```python
from build123d import *

# Parameters (mm, degrees)
F0_W      = 100
F0_H      = 40
F1_DEPTH  = 7
F2_W      = 55
F2_H      = 10
F3_DEPTH  = 8
F4_SIZE   = 3
F5_R      = 2.25
F6_DEPTH  = 18.9
F7_W      = 18
F7_H      = 8
F8_DEPTH  = 3
F9_W      = 55
F9_H      = 10
F10_DEPTH = 1.5
F12_DEPTH = 0.5


# Not quite as in the source:
# - a feature names something its author has since deleted; it is built from what else it names


with BuildPart() as f1:
    # F0 (on Top) → F1 (new body)
    with BuildSketch(Plane.XY):
        with Locations((50, -20)):
            Rectangle(F0_W, F0_H)
    extrude(amount=F1_DEPTH)

    # F2 (on Top) → F3 (cut)
    with BuildSketch(Plane.XY):
        with Locations((50, -20)):
            Rectangle(F2_W, F2_H)
    extrude(amount=F3_DEPTH, mode=Mode.SUBTRACT)

    # F4
    f4_edges = [f1.edges().sort_by_distance(p)[0] for p in [
        (50, -15, 7),
        (22.5, -20, 7),
        (50, -25, 7),
        (77.5, -20, 7),
    ]]
    chamfer(f4_edges, length=F4_SIZE)

    # F5 (on Top) → F6 (cut)
    with BuildSketch(Plane.XY):
        with Locations((12, -35)):
            Circle(F5_R)
        with Locations((31, -35)):
            Circle(F5_R)
        with Locations((50, -35)):
            Circle(F5_R)
        with Locations((69, -35)):
            Circle(F5_R)
        with Locations((88, -35)):
            Circle(F5_R)
        with Locations((95, -28)):
            Circle(F5_R)
        with Locations((95, -12)):
            Circle(F5_R)
        with Locations((88, -5)):
            Circle(F5_R)
        with Locations((69, -5)):
            Circle(F5_R)
        with Locations((50, -5)):
            Circle(F5_R)
        with Locations((31, -5)):
            Circle(F5_R)
        with Locations((12, -5)):
            Circle(F5_R)
        with Locations((5, -12)):
            Circle(F5_R)
        with Locations((5, -28)):
            Circle(F5_R)
    extrude(amount=F6_DEPTH, mode=Mode.SUBTRACT)

    # F7 (on face) → F8 (cut)
    with BuildSketch(Plane(origin=(0, 0, 0), x_dir=(1, 0, 0), z_dir=(0, 0, -1))):
        with Locations((9, 20)):
            Rectangle(F7_W, F7_H)
        with Locations((91, 20)):
            Rectangle(F7_W, F7_H)
    extrude(amount=-F8_DEPTH, mode=Mode.SUBTRACT)

    # F9 (on face) → F10 (cut)
    with BuildSketch(Plane(origin=(0, 0, 0), x_dir=(1, 0, 0), z_dir=(0, 0, -1))):
        Polygon((21, 13.5), (77.5, 13.5), (79, 13.5), (79, 26.5), (21, 26.5), align=None)
        with Locations((50, 20)):
            Rectangle(F9_W, F9_H, mode=Mode.SUBTRACT)
    extrude(amount=-F10_DEPTH, mode=Mode.SUBTRACT)

    # F11 (on face) → F12 (cut)
    with BuildSketch(Plane(origin=(0, 0, 0), x_dir=(1, 0, 0), z_dir=(0, 0, -1))):
        with BuildLine():
            Line((14, 8.5), (16, 8.5))
            Line((16, 8.5), (84, 8.5))
            Line((84, 8.5), (86, 8.5))
            ThreePointArc((86, 8.5), (88.1213203436, 9.3786796564), (89, 11.5))
            Line((89, 11.5), (89, 16))
            Line((89, 16), (87, 16))
            Line((87, 16), (87, 11.5))
            ThreePointArc((87, 11.5), (86.7071067812, 10.7928932188), (86, 10.5))
            Line((86, 10.5), (84, 10.5))
            Line((84, 10.5), (16, 10.5))
            Line((16, 10.5), (14, 10.5))
            ThreePointArc((14, 10.5), (13.2928932188, 10.7928932188), (13, 11.5))
            Line((13, 11.5), (13, 16))
            Line((13, 16), (11, 16))
            Line((11, 16), (11, 11.5))
            ThreePointArc((11, 11.5), (11.8786796564, 9.3786796564), (14, 8.5))
        make_face()
        with BuildLine():
            Line((11, 28.5), (11, 24))
            Line((11, 24), (13, 24))
            Line((13, 24), (13, 28.5))
            ThreePointArc((13, 28.5), (13.2928932188, 29.2071067812), (14, 29.5))
            Line((14, 29.5), (16, 29.5))
            Line((16, 29.5), (84, 29.5))
            Line((84, 29.5), (86, 29.5))
            ThreePointArc((86, 29.5), (86.7071067812, 29.2071067812), (87, 28.5))
            Line((87, 28.5), (87, 24))
            Line((87, 24), (89, 24))
            Line((89, 24), (89, 28.5))
            ThreePointArc((89, 28.5), (88.1213203436, 30.6213203436), (86, 31.5))
            Line((86, 31.5), (84, 31.5))
            Line((84, 31.5), (16, 31.5))
            Line((16, 31.5), (14, 31.5))
            ThreePointArc((14, 31.5), (11.8786796564, 30.6213203436), (11, 28.5))
        make_face()
    extrude(amount=-F12_DEPTH, mode=Mode.SUBTRACT)


solid = f1.part
```
Can you work these out from the model? Positions are in its coordinate system, mm. A direction names the side the tool comes from. Give positions to 0.01 mm unless a question says otherwise; leave off trailing zeros. Loops run counter-clockwise (first coordinate to the right, second up) from the corner with the lowest first, then second, coordinate; pieces in that order, holes last. Notation, with made-up numbers: M 74,64.5 L 100,64.5 A24 ccw 100,90.5 Z; hole C 81.5,49.5 d7. An arc over 180 degrees is marked long. Use one line per item in the form item = value. Start each with the question number.
(1) On a 3-axis mill with a long thin cutter (end or side, diameter ignored), from which of +Z, -Z, +X, -X, +Y, -Y can I reach the whole of each face in a straight line? I mean faces 1 (the flat face through (18, -20, 1)), 2 (the flat face through (49.9, -25.3, 1.5)), 3 (the flat face through (100, -20.3, 3.5)), 4 (the flat face through (50, -15, 3)), 5 (the flat face through (91, -16, 1)). Say none if no direction works.
(2) I want a section at D-D, the plane x = 16. Write out the boundary of the cut face in (y, z), and give its area (3 significant figures).
(3) Thinking about a two-plate mould opening in Y: for faces 6 (the flat face through (0, -20.3, 3.5)), 7 (the flat face through (49, 0, 3)), 8 (the cylindrical face through (48.34, -33.48, 3.45)), which applies, released by +Y, released by -Y, zero draft, split by the parting line, or undercut?
(4) I want a section at C-C, the plane z = 5. State how many separate pieces and enclosed holes the cut face has, and give its area (3 significant figures).
(5) Please list where these lines run through material, in increasing order: line 1 (X direction, y = -5, z = 3.75); line 2 (Y direction, x = 88, z = 5.5); line 3 (Y direction, x = 88, z = 2.5).
(6) I want a section at A-A, the plane x = 60. Write out the boundary of the cut face in (y, z).
(7) I want a section at B-B, the plane y = -5. Write out the boundary of the cut face in (x, z), and give its area (4 significant figures).
(8) I'm going to push flat-ended pins straight in: P1, Ø6.5, axis at x = 42.5, y = -23, coming from the -Z side; P2, Ø1.5, axis at y = -20.5, z = 1.5, coming from the +X side. Where does each tip first touch, or does it pass through?
Worked out:
q1.face_1 = -Z, -X
q1.face_2 = -Z
q1.face_3 = +Z, -Z, +X, +Y, -Y
q1.face_4 = +Z, -Z
q1.face_5 = -Z, +X
q2.outline = M -40,0 L -31.5,0 L -31.5,0.5 L -29.5,0.5 L -29.5,0 L -24,0 L -24,3 L -16,3 L -16,0 L -10.5,0 L -10.5,0.5 L -8.5,0.5 L -8.5,0 L 0,0 L 0,7 L -40,7 Z
q2.area = 254 mm²
q3.face_6 = zero draft
q3.face_7 = released by +Y
q3.face_8 = undercut
q4.separate_pieces = 1
q4.enclosed_holes = 15
q4.area = 3,090 mm²
q5.line_1 = 0 to 9.75, 14.25 to 28.75, 33.25 to 47.75, 52.25 to 66.75, 71.25 to 85.75, 90.25 to 100
q5.line_2 = -40 to -37.25, -32.75 to -7.25, -2.75 to 0
q5.line_3 = -40 to -37.25, -32.75 to -24, -16 to -7.25, -2.75 to 0
q6.outline = M -40,0 L -31.5,0 L -31.5,0.5 L -29.5,0.5 L -29.5,0 L -26.5,0 L -26.5,1.5 L -25,1.5 L -25,4 L -28,7 L -40,7 Z; M -15,1.5 L -13.5,1.5 L -13.5,0 L -10.5,0 L -10.5,0.5 L -8.5,0.5 L -8.5,0 L 0,0 L 0,7 L -12,7 L -15,4 Z
q7.outline = M 0,0 L 9.75,0 L 9.75,7 L 0,7 Z; M 14.25,0 L 28.75,0 L 28.75,7 L 14.25,7 Z; M 33.25,0 L 47.75,0 L 47.75,7 L 33.25,7 Z; M 52.25,0 L 66.75,0 L 66.75,7 L 52.25,7 Z; M 71.25,0 L 85.75,0 L 85.75,7 L 71.25,7 Z; M 90.25,0 L 100,0 L 100,7 L 90.25,7 Z
q7.area = 542.5 mm²
q8.P1 = 1.5
q8.P2 = 82
